Could you check a few things on this model? Use its own coordinates, in mm. Face numbers are marked on the shaded views. A direction names the side the tool comes from. Round coordinates to 2 decimals unless told otherwise and drop trailing zeros. Loops run counter-clockwise (first coordinate to the right, second up) from the corner with the lowest first, then second, coordinate; pieces in that order, holes last. Notation, with made-up numbers: (-3, 22.25) - (33, 22.25) arc R17 cw to (33, 54.25) - close; hole circle Ø9 at (25, 10). An arc over 180 degrees is marked (long way). Answer as CSV lines item,"result". Start each with the question number.
1) Suppose I cut it at A-A, the plane x = 1.25. Write out the boundary of the cut face in (y, z), then the cut area to 3 significant figures.
2) Please list where these lines run through material, in increasing order: line 1 along Y through (x, z) = (-11.5, 0.25); line 2 along X through (y, z) = (3.2, -0.5); line 3 along Y through (x, z) = (-2.25, 1.5).
3) Which directions (+Z, -Z, +X, -X, +Y, -Y) give clear straight access to the entire face, cutting with the end or side of a thin tool? Please do the marked faces 1 and 2.
4) Suppose I cut it at B-B, the plane z = -3.25. Write out the boundary of the cut face in (x, y).
5) Suppose I cut it at C-C, the plane x = 10. Write out the boundary of the cut face in (y, z).
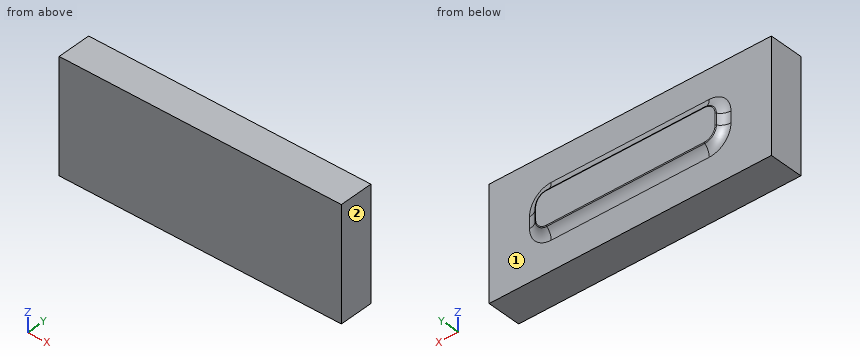
```python
from build123d import *

# Parameters (mm, degrees)
SKETCH_1_W      = 25
SKETCH_1_H      = 10
EXTRUDE_1_DEPTH = 3
EXTRUDE_2_DEPTH = 0.5
FILLET_1_R      = 1.1
FILLET_2_R      = 0.1


with BuildPart() as part:
    # 草图1 → 凸台-拉伸1 (new body)
    with BuildSketch(Plane(origin=(0, 0, 0), x_dir=(1, 0, 0), z_dir=(0, 1, 0))):
        Rectangle(SKETCH_1_W, SKETCH_1_H)
    extrude(amount=EXTRUDE_1_DEPTH)

    # 草图2 → 凸台-拉伸2 (add)
    with BuildSketch(Plane(origin=(0, 3, 0), x_dir=(1, 0, 0), z_dir=(0, 1, 0))):
        with BuildLine():
            Line((7, 1.5), (-7, 1.5))
            ThreePointArc((-7, 1.5), (-7.707106781, 1.207106781), (-8, 0.5))
            Line((-8, 0.5), (-8, -0.5))
            ThreePointArc((-8, -0.5), (-7.707106781, -1.207106781), (-7, -1.5))
            Line((-7, -1.5), (7, -1.5))
            ThreePointArc((7, -1.5), (7.707106781, -1.207106781), (8, -0.5))
            Line((8, -0.5), (8, 0.5))
            ThreePointArc((8, 0.5), (7.707106781, 1.207106781), (7, 1.5))
        make_face()
    extrude(amount=EXTRUDE_2_DEPTH)

    # 圆角1
    # the kernel refuses this fillet: 1.1 mm, written as the material it adds along each edge
    with BuildSketch(Plane(origin=(-7, 3, 0.5), x_dir=(-1, 0, 0), z_dir=(0, 0, -1))) as fillet_1_piece_1:
        with BuildLine():
            CenterArc((1.921954446, 1.1), FILLET_1_R, 213.055731151, 56.944268849)
            Line((1, 0.5), (0.981560911, 0.488))
            ThreePointArc((0.981560911, 0.488), (0.978, 0.25), (0.978, 0))
            Line((0.978, 0), (1, -0.022))
            Line((1, -0.022), (1.921954446, -0.022))
            Line((1.921954446, -0.022), (1.921954446, 0))
        make_face()
    revolve(axis=Axis((-7, 3, 0.5), (0, 1, 0)), revolution_arc=90)
    with BuildSketch(Plane(origin=(-8, 3, -0.5), x_dir=(-1, 0, 0), z_dir=(0, 0, 1)), Plane(origin=(8, 3, 0.5), x_dir=(1, 0, 0), z_dir=(0, 0, -1))) as fillet_1_piece_2:
        with BuildLine():
            CenterArc((0.921954446, -1.1), FILLET_1_R, 90, 56.944268849)
            Line((0, -0.5), (-0.018439089, -0.488))
            ThreePointArc((-0.018439089, -0.488), (-0.022, -0.25), (-0.022, 0))
            Line((-0.022, 0), (0, 0.022))
            Line((0, 0.022), (0.921954446, 0.022))
            Line((0.921954446, 0.022), (0.921954446, 0))
        make_face()
    extrude(amount=1)
    with BuildSketch(Plane(origin=(-7, 3, -0.5), x_dir=(0, 0, -1), z_dir=(1, 0, 0))) as fillet_1_piece_3:
        with BuildLine():
            CenterArc((1.921954446, 1.1), FILLET_1_R, 213.055731151, 56.944268849)
            Line((1, 0.5), (0.981560911, 0.488))
            ThreePointArc((0.981560911, 0.488), (0.978, 0.25), (0.978, 0))
            Line((0.978, 0), (1, -0.022))
            Line((1, -0.022), (1.921954446, -0.022))
            Line((1.921954446, -0.022), (1.921954446, 0))
        make_face()
    revolve(axis=Axis((-7, 3, -0.5), (0, 1, 0)), revolution_arc=90)
    with BuildSketch(Plane(origin=(7, 3, -1.5), x_dir=(0, 0, -1), z_dir=(-1, 0, 0)), Plane(origin=(-7, 3, 1.5), x_dir=(0, 0, 1), z_dir=(1, 0, 0))) as fillet_1_piece_4:
        with BuildLine():
            CenterArc((0.921954446, -1.1), FILLET_1_R, 90, 56.944268849)
            Line((0, -0.5), (-0.018439089, -0.488))
            ThreePointArc((-0.018439089, -0.488), (-0.022, -0.25), (-0.022, 0))
            Line((-0.022, 0), (0, 0.022))
            Line((0, 0.022), (0.921954446, 0.022))
            Line((0.921954446, 0.022), (0.921954446, 0))
        make_face()
    extrude(amount=14)
    with BuildSketch(Plane(origin=(7, 3, -0.5), x_dir=(1, 0, 0), z_dir=(0, 0, 1))) as fillet_1_piece_5:
        with BuildLine():
            CenterArc((1.921954446, 1.1), FILLET_1_R, 213.055731151, 56.944268849)
            Line((1, 0.5), (0.981560911, 0.488))
            ThreePointArc((0.981560911, 0.488), (0.978, 0.25), (0.978, 0))
            Line((0.978, 0), (1, -0.022))
            Line((1, -0.022), (1.921954446, -0.022))
            Line((1.921954446, -0.022), (1.921954446, 0))
        make_face()
    revolve(axis=Axis((7, 3, -0.5), (0, 1, 0)), revolution_arc=90)
    with BuildSketch(Plane(origin=(7, 3, 0.5), x_dir=(0, 0, 1), z_dir=(-1, 0, 0))) as fillet_1_piece_6:
        with BuildLine():
            CenterArc((1.921954446, 1.1), FILLET_1_R, 213.055731151, 56.944268849)
            Line((1, 0.5), (0.981560911, 0.488))
            ThreePointArc((0.981560911, 0.488), (0.978, 0.25), (0.978, 0))
            Line((0.978, 0), (1, -0.022))
            Line((1, -0.022), (1.921954446, -0.022))
            Line((1.921954446, -0.022), (1.921954446, 0))
        make_face()
    revolve(axis=Axis((7, 3, 0.5), (0, 1, 0)), revolution_arc=90)

    # 圆角2
    fillet_2_edges = [part.edges().sort_by_distance(p)[0] for p in [
        (-7.707106781, 3.5, 1.207106781),
        (0, 3.5, 1.5),
        (7.707106781, 3.5, 1.207106781),
        (8, 3.5, 0),
        (7.707106781, 3.5, -1.207106781),
        (0, 3.5, -1.5),
        (-7.707106781, 3.5, -1.207106781),
        (-8, 3.5, 0),
    ]]
    fillet(fillet_2_edges, radius=FILLET_2_R)


solid = part.part
```
Filled sheet:
1,outline,"(0, -5) - (3, -5) - (3, -2.42) arc R1.1 cw to (3.46, -1.53) arc R0.1 ccw to (3.5, -1.45) - (3.5, 1.45) arc R0.1 ccw to (3.46, 1.53) arc R1.1 cw to (3, 2.42) - (3, 5) - (0, 5) - close"
1,area,"31.8 mm²"
2,line 1,"0 to 3"
2,line 2,"-8.29 to 8.29"
2,line 3,"0 to 3.48"
3,face 1,"+Y"
3,face 2,"+Z, -Z, +X, +Y, -Y"
4,outline,"(-12.5, 0) - (12.5, 0) - (12.5, 3) - (-12.5, 3) - close"
5,outline,"(0, -5) - (3, -5) - (3, 5) - (0, 5) - close"
